from build123d import *

# Parameters (mm, degrees)
F1_DEPTH      = 120
F0_W          = 5
F0_H          = 5
F2_DEPTH      = 120
F2_DEPTH_BACK = 20
F6_R          = 12.5
F6_R_2        = 10
F7_DEPTH      = 30
F8_R          = 10
F9_DEPTH      = 25
F8_W          = 42
F8_H          = 42
F8_W_2        = 40
F8_H_2        = 40
F10_DEPTH     = 10
F11_DEPTH     = 25
F12_W         = 40
F12_H         = 30
F12_R         = 2.4384
F13_DEPTH     = 25
F16_R         = 15
F16_R_2       = 10
F17_DEPTH     = 2
F18_R         = 0.99999
F19_SIZE      = 1


# Not quite as in the source:
# - a fillet or chamfer is up to 0.001 mm smaller than in the source, because OpenCascade refuses the exact size
# - a feature of the source that left no trace in its solid (it failed there, or was rolled back) is left out
# - a feature names something its author has since deleted; it is built from what else it names


with BuildPart() as f1:
    # F0 (on Front) → F1 (new body)
    with BuildSketch(Plane.XZ):
        with BuildLine():
            ThreePointArc((-22.5, -40), (-39.6160493738, -23.1693468188), (-45.8938993767, 0))
            Line((-45.8938993767, 0), (-50.8938993767, 0))
            ThreePointArc((-50.8938993767, 0), (-45.7803505669, -22.233949171), (-31.4672686099, -40))
            Line((-31.4672686099, -40), (-22.5, -40))
        make_face()
        with BuildLine():
            Line((50.8938993767, 0), (45.8938993767, 0))
            ThreePointArc((45.8938993767, 0), (39.6160493738, -23.1693468188), (22.5, -40))
            Line((22.5, -40), (31.4672686099, -40))
            ThreePointArc((31.4672686099, -40), (45.7803505669, -22.233949171), (50.8938993767, 0))
        make_face()
        with BuildLine():
            ThreePointArc((-45.8938993767, 0), (0, 45.8938993767), (45.8938993767, 0))
            Line((45.8938993767, 0), (50.8938993767, 0))
            ThreePointArc((50.8938993767, 0), (0, 50.8938993767), (-50.8938993767, 0))
            Line((-50.8938993767, 0), (-45.8938993767, 0))
        make_face()
    extrude(amount=F1_DEPTH)

    # F0 (on Front) → F2 (join, two sides)
    with BuildSketch(Plane.XZ) as f2_sk:
        with BuildLine():
            Line((31.4672686099, -40), (22.5, -40))
            ThreePointArc((22.5, -40), (15.954031767, -43.0316031583), (9.0138781887, -45))
            Line((9.0138781887, -45), (23.7737038294, -45))
            ThreePointArc((23.7737038294, -45), (27.7333960958, -42.6737358894), (31.4672686099, -40))
        make_face()
        with BuildLine():
            ThreePointArc((9.0138781887, -45), (15.954031767, -43.0316031583), (22.5, -40))
            Line((22.5, -40), (0, -40))
            Line((0, -40), (-22.5, -40))
            ThreePointArc((-22.5, -40), (-15.954031767, -43.0316031583), (-9.0138781887, -45))
            Line((-9.0138781887, -45), (9.0138781887, -45))
        make_face()
        with BuildLine():
            ThreePointArc((-9.0138781887, -45), (-15.954031767, -43.0316031583), (-22.5, -40))
            Line((-22.5, -40), (-31.4672686099, -40))
            ThreePointArc((-31.4672686099, -40), (-27.7333960958, -42.6737358894), (-23.7737038294, -45))
            Line((-23.7737038294, -45), (-9.0138781887, -45))
        make_face()
        with BuildLine():
            ThreePointArc((-23.7737038294, -45), (-27.7333960958, -42.6737358894), (-31.4672686099, -40))
            Line((-31.4672686099, -40), (-55, -40))
            Line((-55, -40), (-55, -65))
            Line((-55, -65), (-50, -65))
            Line((-50, -65), (-50, -45))
            Line((-50, -45), (-23.7737038294, -45))
        make_face()
        with Locations((-52.5, -67.5)):
            Rectangle(F0_W, F0_H)
        with BuildLine():
            Line((55, -40), (31.4672686099, -40))
            ThreePointArc((31.4672686099, -40), (27.7333960958, -42.6737358894), (23.7737038294, -45))
            Line((23.7737038294, -45), (50, -45))
            Line((50, -45), (50, -65))
            Line((50, -65), (-50, -65))
            Line((-50, -65), (-50, -70))
            Line((-50, -70), (55, -70))
            Line((55, -70), (55, -40))
        make_face()
    extrude(amount=F2_DEPTH)
    extrude(f2_sk.sketch, amount=-F2_DEPTH_BACK)

    # F6 (on offset) → F7 (join)
    with BuildSketch(Plane.XY.offset(76)):
        with Locations((0, -15)):
            Circle(F6_R)
        with Locations((0, -15)):
            Circle(F6_R_2, mode=Mode.SUBTRACT)
    extrude(amount=-F7_DEPTH)

    # F8 (on offset) → F9 (cut)
    with BuildSketch(Plane.XY.offset(56)):
        with Locations((0, -15)):
            Circle(F8_R)
    extrude(amount=-F9_DEPTH, mode=Mode.SUBTRACT)

    # F8 (on offset) → F10 (join)
    with BuildSketch(Plane.XY.offset(56)):
        with Locations((0, -66)):
            Rectangle(F8_W, F8_H)
        with Locations((0, -66)):
            Rectangle(F8_W_2, F8_H_2, mode=Mode.SUBTRACT)
    extrude(amount=-F10_DEPTH)

    # F8 (on offset) → F11 (cut)
    with BuildSketch(Plane.XY.offset(56)):
        with Locations((0, -66)):
            Rectangle(F8_W_2, F8_H_2)
    extrude(amount=-F11_DEPTH, mode=Mode.SUBTRACT)

    # F12 (on face) → F13 (cut)
    with BuildSketch(Plane.XY.offset(-40)):
        with Locations((3.8294e-06, 35)):
            Rectangle(F12_W, F12_H)
        with Locations((0, 60)):
            Circle(F12_R)
    extrude(amount=-F13_DEPTH, mode=Mode.SUBTRACT)

    # F16 (on offset) → F17 (join)
    with BuildSketch(Plane.XY.offset(68.5)):
        with Locations((0, -15)):
            Circle(F16_R)
        with Locations((0, -15)):
            Circle(F16_R_2, mode=Mode.SUBTRACT)
    extrude(amount=F17_DEPTH)

    # F18 (radius 1 in the source; OpenCascade refuses exactly that, so slightly less here)
    f18_edges = [f1.edges().sort_by_distance(p)[0] for p in [
        (-15, -15, 70.5),
        (-15, -15, 68.5),
        (-12.5, -15, 76),
    ]]
    fillet(f18_edges, radius=F18_R)

    # F19
    f19_edges = [f1.edges().sort_by_distance(p)[0] for p in [
        (-10, -15, 76),
    ]]
    chamfer(f19_edges, length=F19_SIZE)


solid = f1.part
Check sheet for the modelled part. Datum: model origin and axes. Units: mm. A direction names the side the tool comes from. Give positions to 0.01 mm unless a question says otherwise; leave off trailing zeros. Loops run counter-clockwise (first coordinate to the right, second up) from the corner with the lowest first, then second, coordinate; pieces in that order, holes last. Notation, with made-up numbers: M 84.5,2 L 115.5,2 A20 ccw 115.5,23 Z; hole C -38,28.5 d11. An arc over 180 degrees is marked long. Return JSON: item names as keys, results as strings. Group by question number.
1. Cross-section at A-A on z = -53. Record the boundary of the cut face in (x, y).
2. Thickness scan on L1, parallel to Y at x = 0, z = 55.75; L2, parallel to Y at x = 0, z = 47.5; L3, parallel to Z at x = -49.5, y = 12.5. Record the ranges inside material, lowest first.
3. Tool access check on faces 1 (the flat face through (50, -51, -55)), 2 (the flat face through (-5.3, -3.5, 68.5)), 3 (the cylindrical face through (-2.71, -27.203, 72.782)), 4 (the flat face through (21, -66, 51)), 5 (the flat face through (-21, -66, 51)). Record the directions out of +Z, -Z, +X, -X, +Y, -Y that give a thin tool (end or side, any length) a straight path to the whole face; none if there is none.
4. Go/stop test with flat-tipped pins: pin 1 (8 mm diameter, centred on x = 40, y = -37, fed in from +Z); pin 2 (6 mm diameter, centred on y = -56.5, z = -11, fed in from -X); pin 3 (12 mm diameter, centred on x = -2.5, y = 5, fed in from +Z). Record where each tip stops, or that it passes through.
5. Mould release check, pull along Z, two halves, no side actions. Record for faces 6 (the flat face through (-5.3, -3.5, 70.5)), 7 (the flat face through (-1, -51, -45)), 8 (the flat face through (-50, -51, -55)), 9 (the flat face through (-20, -66, 49)): released by +Z, released by -Z, zero draft, split by the parting line, or undercut.
6. Cross-section at C-C on x = -40.5. Record the boundary of the cut face in (y, z), plus the area to 3 significant figures.
7. Cross-section at B-B on y = 7. Record the boundary of the cut face in (x, z).
8. Cross-section at D-D on y = -110. Record the boundary of the cut face in (x, z), plus the area to 3 significant figures.
Return value:
{
 "1": {"outline": "M -55,-120 L -50,-120 L -50,20 L -55,20 Z; M 50,-120 L 55,-120 L 55,20 L 50,20 Z"},
 "2": {"L1": "-87 to -86, -46 to -45, -27.5 to -25, -5 to -2.5", "L2": "-120 to -86, -46 to -25, -5 to 0", "L3": "-70 to -65, -45 to -40"},
 "3": {"face 1": "+Y, -Y", "face 2": "none", "face 3": "+Z", "face 4": "+Z, +X, +Y, -Y", "face 5": "+Z, -X, +Y, -Y"},
 "4": {"pin 1": "z = 35.97", "pin 2": "x = -50.26", "pin 3": "z = 70.49"},
 "5": {"face 6": "released by +Z", "face 7": "undercut", "face 8": "undercut", "face 9": "zero draft"},
 "6": {"outline": "M -120,-70 L 20,-70 L 20,-65 L -120,-65 Z; M -120,-45 L 20,-45 L 20,-40 L -120,-40 Z; M -120,-30.82 L 0,-30.82 L 0,-21.59 L -120,-21.59 Z; M -120,21.59 L 0,21.59 L 0,30.82 L -120,30.82 Z", "area": "3,620 mm^2"},
 "7": {"outline": "M -55,-70 L 55,-70 L 55,-40 L -55,-40 Z; hole M -50,-65 L 50,-65 L 50,-45 L -50,-45 Z"},
 "8": {"outline": "M -55,-70 L 55,-70 L 55,-40 L 31.47,-40 A50.89 ccw long -31.47,-40 L -55,-40 Z; hole M -50,-65 L 50,-65 L 50,-45 L -50,-45 Z; hole M -22.5,-40 L 22.5,-40 A45.89 ccw long Z", "area": "2,530 mm^2"}
}
